Autodesk Inventor part; units mm, degrees
ref_plane "YZ Plane" through (0, 0, 0) normal (1, 0, 0) x (0, 1, 0)
ref_plane "XZ Plane" through (0, 0, 0) normal (0, 1, 0) x (-1, 0, 0)
ref_plane "XY Plane" through (0, 0, 0) normal (0, 0, 1) x (1, 0, 0)
sketch "Sketch1" plane through (0, 0, 0) normal (0, 0, 1) x (1, 0, 0)
  arc A0 (-183.6588, -17.77) -> (-179.4288, -22) centre (-179.4288, -17.77) ccw
  arc A1 (-179.9924, 22) -> (-183.6588, 16.912) centre (-179.5223, 17.7962) ccw
  line L0 (-183.6588, -17.77) -> (-183.6588, 16.912)
  line L1 (-205.2488, 21.796) -> (-205.2488, -22.654)
  line L2 (-286.5288, 24.971) -> (-208.4238, 24.971)
  line L3 (-286.5288, -25.829) -> (-208.4238, -25.829)
  line L4 (-52.9925, -22) -> (-179.4288, -22)
  line L5 (-52.4305, 22) -> (-179.9924, 22)
  arc A2 (-48.2588, 16.912) -> (-52.4305, 22) centre (-52.4009, 17.7701) ccw
  line L6 (-48.2588, -17.77) -> (-48.2588, 16.912)
  arc A3 (-52.9925, -22) -> (-48.2588, -17.77) centre (-52.4887, -17.8001) ccw
  arc A4 (-205.2488, 21.796) -> (-208.4238, 24.971) centre (-208.4238, 21.796) ccw
  arc A5 (-208.4238, -25.829) -> (-205.2488, -22.654) centre (-208.4238, -22.654) ccw
  line L7 (204.3262, -25.4) -> (282.4312, -25.4)
  line L8 (204.3262, 25.4) -> (282.4312, 25.4)
  line L9 (44.1612, -17.77) -> (44.1612, 16.912)
  arc A6 (44.1612, -17.77) -> (48.3912, -22) centre (48.3912, -17.77) ccw
  line L10 (175.3896, 22) -> (47.8276, 22)
  line L11 (174.8276, -22) -> (48.3912, -22)
  arc A7 (174.8276, -22) -> (179.5612, -17.77) centre (175.3313, -17.8001) ccw
  arc A8 (179.5612, 16.912) -> (175.3896, 22) centre (175.4192, 17.7701) ccw
  arc A9 (47.8276, 22) -> (44.1612, 16.912) centre (48.2978, 17.7962) ccw
  line L12 (179.5612, -17.77) -> (179.5612, 16.912)
  arc A10 (201.1512, -22.225) -> (204.3262, -25.4) centre (204.3262, -22.225) ccw
  arc A11 (204.3262, 25.4) -> (201.1512, 22.225) centre (204.3262, 22.225) ccw
  line L13 (201.1512, 22.225) -> (201.1512, -22.225)
  line L14 (-286.5288, 38.1) -> (282.4312, 38.1)
  line L15 (-286.5288, -38.1) -> (282.4312, -38.1)
  line L16 (282.4312, 38.1) -> (282.4312, 25.4)
  line L17 (282.4312, -25.4) -> (282.4312, -38.1)
  line L18 (-286.5288, 38.1) -> (-286.5288, 24.971)
  line L19 (-286.5288, -25.829) -> (-286.5288, -38.1)
  point P0 (0, 0)
  dimension "d0" = 135.4
  dimension "d1" = 44
  dimension "d2" = 78.105
  dimension "d3" = 50.8
  dimension "d4" = 44.45
  dimension "d5" = 21.59
  dimension "d6" = 135.4
  dimension "d7" = 44
  dimension "d8" = 78.105
  dimension "d9" = 50.8
  dimension "d10" = 568.96
  dimension "d11" = 21.59
extrude "Extrusion1" add sketch "Sketch1" along normal blind 9.525
sketch "Sketch2" plane through (-286.5288, 38.1, 0) normal (0, 1, 0) x (1, 0, 0)
  line L0 (0, 57.15) -> (568.96, 57.15)
  line L1 (568.96, 57.15) -> (568.96, 0)
  line L2 (568.96, 0) -> (0, 0)
  line L3 (0, 0) -> (0, 57.15)
  circle A0 centre (40.64, 28.575) radius 13
  circle A1 centre (140.776, 28.575) radius 13
  circle A2 centre (230.152, 28.575) radius 16
  circle A3 centre (528.32, 28.575) radius 13
  circle A4 centre (428.184, 28.575) radius 13
  circle A5 centre (338.808, 28.575) radius 16
  point P0 (286.5288, 0)
  point P1 (99.06, 38.1)
  dimension "d14" = 26
  dimension "d15" = 26
  dimension "d16" = 32
  dimension "d17" = 26
  dimension "d18" = 26
  dimension "d19" = 32
  dimension "d20" = 568.96
  dimension "d21" = 57.15
  dimension "d22" = 40.64
  dimension "d23" = 140.776
  dimension "d24" = 230.152
  dimension "d25" = 230.152
  dimension "d26" = 40.64
  dimension "d27" = 140.776
extrude "Extrusion2" add sketch "Sketch2" against normal blind 9.525
sketch "Sketch3" plane through (-286.5288, -38.1, 0) normal (0, -1, 0) x (1, 0, 0)
  line L0 (0, 0) -> (568.96, 0)
  line L1 (568.96, 0) -> (568.96, -57.15)
  line L2 (568.96, -57.15) -> (0, -57.15)
  line L3 (0, -57.15) -> (0, 0)
  circle A0 centre (40.64, -28.575) radius 13
  circle A1 centre (140.776, -28.575) radius 13
  circle A2 centre (230.152, -28.575) radius 16
  circle A3 centre (528.32, -28.575) radius 13
  circle A4 centre (428.184, -28.575) radius 13
  circle A5 centre (338.808, -28.575) radius 16
  point P0 (286.5288, 0)
  dimension "d30" = 26
  dimension "d31" = 26
  dimension "d32" = 32
  dimension "d33" = 26
  dimension "d34" = 26
  dimension "d35" = 32
  dimension "d36" = 568.96
  dimension "d37" = 57.15
  dimension "d38" = 40.64
  dimension "d39" = 140.776
  dimension "d40" = 230.152
  dimension "d41" = 230.152
  dimension "d42" = 40.64
  dimension "d43" = 140.776
extrude "Extrusion3" add sketch "Sketch3" against normal blind 9.525
sketch "Sketch5" plane through (282.4312, -38.1, -57.15) normal (0, 0, -1) x (-1, 0, 0)
  arc A0 (102.8699, 20.33) -> (107.0999, 16.1) centre (107.0999, 20.33) ccw
  arc A1 (106.5363, 60.1) -> (102.8699, 55.012) centre (107.0065, 55.8962) ccw
  line L0 (102.8699, 20.33) -> (102.8699, 55.012)
  line L1 (81.2799, 59.896) -> (81.2799, 15.446)
  line L2 (-0.0001, 63.071) -> (78.1049, 63.071)
  line L3 (0, 12.271) -> (78.105, 12.271)
  line L4 (233.5363, 16.1) -> (107.0999, 16.1)
  line L5 (234.0983, 60.1) -> (106.5363, 60.1)
  arc A2 (238.2699, 55.012) -> (234.0983, 60.1) centre (234.1279, 55.8701) ccw
  line L6 (238.2699, 20.33) -> (238.2699, 55.012)
  arc A3 (233.5363, 16.1) -> (238.2699, 20.33) centre (234.04, 20.2999) ccw
  arc A4 (81.2799, 59.896) -> (78.1049, 63.071) centre (78.1049, 59.896) ccw
  arc A5 (78.105, 12.271) -> (81.2799, 15.446) centre (78.1049, 15.446) ccw
  line L7 (490.855, 12.7) -> (568.96, 12.7)
  line L8 (490.855, 63.5) -> (568.9599, 63.5)
  line L9 (330.69, 20.33) -> (330.69, 55.012)
  arc A6 (330.69, 20.33) -> (334.92, 16.1) centre (334.92, 20.33) ccw
  line L10 (461.9184, 60.1) -> (334.3564, 60.1)
  line L11 (461.3564, 16.1) -> (334.92, 16.1)
  arc A7 (461.3564, 16.1) -> (466.09, 20.33) centre (461.8601, 20.2999) ccw
  arc A8 (466.09, 55.012) -> (461.9184, 60.1) centre (461.948, 55.8701) ccw
  arc A9 (334.3564, 60.1) -> (330.69, 55.012) centre (334.8266, 55.8962) ccw
  line L12 (466.09, 20.33) -> (466.09, 55.012)
  arc A10 (487.68, 15.875) -> (490.855, 12.7) centre (490.855, 15.875) ccw
  arc A11 (490.855, 63.5) -> (487.68, 60.325) centre (490.855, 60.325) ccw
  line L13 (487.68, 60.325) -> (487.68, 15.875)
  line L14 (-0.0001, 76.2) -> (568.9599, 76.2)
  line L15 (0, 0) -> (568.96, 0)
  line L16 (568.9599, 76.2) -> (568.9599, 63.5)
  line L17 (568.96, 12.7) -> (568.96, 0)
  line L18 (-0.0001, 76.2) -> (-0.0001, 63.071)
  line L19 (0, 12.271) -> (0, 0)
  point P0 (282.4312, 38.1)
  dimension "d60" = 135.4
  dimension "d61" = 44
  dimension "d62" = 78.105
  dimension "d63" = 50.8
  dimension "d64" = 44.45
  dimension "d65" = 21.59
  dimension "d66" = 135.4
  dimension "d67" = 44
  dimension "d68" = 78.105
  dimension "d69" = 50.8
  dimension "d70" = 568.96
  dimension "d71" = 21.59
extrude "Extrusion5" add sketch "Sketch5" along normal blind 9.525
sketch "Sketch6" plane through (282.4313, 24.971, -57.15) normal (1, 0, 0) x (0, 0, -1)
  point P0 (-57.15, -24.971)
properties part number "BT-BTK120-DriveFrameTube" material "Aluminum 6061"
Geometry: final body of the model. Coordinates: model frame, mm. A direction names the side the tool comes from. Round coordinates to 2 decimals unless told otherwise and drop trailing zeros. Order: outer loops, then holes, each group sorted by start corner. A loop starts at its lowest first (then second) coordinate and runs counter-clockwise, first axis right, second up. Notation, with made-up numbers: (81.25, 67) - (100.25, 67) arc R14 cw to (100.25, 82) - close; hole circle Ø5 at (-0.5, 30). An arc over 180 degrees is marked (long way). Write each question's results on one line, items separated by ' | '.
Item 1: Mould query, pull axis X, two halves, no side actions, for faces 1 (the flat face through (-286.529, 32, -62)), 2 (the flat face through (-48.259, -1, -62)), 3 (the flat face through (2, 5, -57.15)). Classes: pulls with the +X half, pulls with the -X half, needs draft (parallel to the pull), parting line crosses it, or undercut.
Completed:
face 1: pulls with the -X half | face 2: undercut | face 3: needs draft
Item 2: Section B-B, the plane y = -13. Return the cut outline in (x, z) (3 decimals), and give its area (3 significant figures).
Completed:
outline: (-205.249, -66.675) - (-183.659, -66.675) - (-183.659, -57.15) - (-205.249, -57.15) - close; (-205.249, 0) - (-183.659, 0) - (-183.659, 9.525) - (-205.249, 9.525) - close; (-48.259, -66.675) - (44.161, -66.675) - (44.161, -57.15) - (-48.259, -57.15) - close; (-48.259, 0) - (44.161, 0) - (44.161, 9.525) - (-48.259, 9.525) - close; (179.561, -66.675) - (201.151, -66.675) - (201.151, -57.15) - (179.561, -57.15) - close; (179.561, 0) - (201.151, 0) - (201.151, 9.525) - (179.561, 9.525) - close | area: 2,580 mm^2
Item 3: First-contact query: pin 1 Ø23.5 at (x, z) = (141.66, -28.58) entering from -Y; pin 2 Ø3 at (y, z) = (-4.5, 5.5) entering from -X. Flat tips, straight axial feed; report the tip coordinate or a pass-through.
Completed:
pin 1: through | pin 2: x = -205.25
Item 4: Section A-A, the plane x = -78. Return the cut outline in (y, z) (3 decimals), and give its area (3 significant figures).
Completed:
outline: (-38.1, -66.675) - (-22, -66.675) - (-22, -57.15) - (-28.575, -57.15) - (-28.575, 0) - (-22, 0) - (-22, 9.525) - (-38.1, 9.525) - close; (22, -66.675) - (38.1, -66.675) - (38.1, 9.525) - (22, 9.525) - (22, 0) - (28.575, 0) - (28.575, -57.15) - (22, -57.15) - close | area: 1,700 mm^2
Item 5: Section C-C, the plane x = 30. Return the cut outline in (y, z) (3 decimals), and give its area (3 significant figures).
Completed:
outline: (-38.1, -66.675) - (38.1, -66.675) - (38.1, 9.525) - (-38.1, 9.525) - close; hole (-28.575, -57.15) - (28.575, -57.15) - (28.575, 0) - (-28.575, 0) - close | area: 2,540 mm^2
Item 6: Material intervals for line 1 along Z through (x, y) = (-222, -27.5) (3 decimals); line 2 along Y through (x, z) = (-189, -51) (3 decimals); line 3 along X through (y, z) = (-17.5, 2), sorted ascending. Write a range as [from, to].
Completed:
line 1: [-66.675, -57.15], [0, 9.525] | line 2: [-38.1, -28.575], [28.575, 38.1] | line 3: [-205.25, -183.66], [-48.26, 44.16], [179.56, 201.15]
Item 7: Reachability of faces 4 (the flat face through (-205.249, 0, -62)), 5 (the flat face through (-6, 0, 0)), 6 (the flat face through (44.161, -1, 5)) from +Z, -Z, +X, -X, +Y, -Y: full face, straight path, thin tool, end or side. Return the list, or none.
Completed:
face 4: +Z, -Z, -X | face 5: +X, -X | face 6: +Z, -Z
